Build history of the part. All positions in model axes, mm. A direction names the side the tool comes from. Give positions to 0.01 mm unless a question says otherwise; leave off trailing zeros. Write each loop counter-clockwise with the first axis right and the second up, starting at its lowest first coordinate (ties: lowest second). Pieces come first, ordered by that corner, then holes. Notation, with made-up numbers: (79, 47.5) -> (106, 47.5) arc R21 cw to (106, 59.5) -> close; hole circle Ø4 at (48, -3.75). An arc over 180 degrees is marked (long way). Put each result on its own line as item: value.
from build123d import *

# Parameters (mm, degrees)
F0_R      = 41
F0_R_2    = 8
F2_DEPTH  = 5
F5_DEPTH  = 5.001
F7_DEPTH  = 5.001
F9_DEPTH  = 5.001
F11_DEPTH = 5.001
F13_DEPTH = 5.001
F15_DEPTH = 25
F16_R     = 8
F17_DEPTH = 5.001
F19_DEPTH = 5.001
F21_DEPTH = 5.001
F22_R     = 8
F23_DEPTH = 5.001
F24_R     = 8
F25_DEPTH = 5.001
F26_R     = 8
F27_DEPTH = 5.001
F28_R     = 19.931343
F29_DEPTH = 5.001
F30_R     = 19.962779
F31_DEPTH = 5.001
F32_R     = 19.962779
F33_DEPTH = 5.001
F34_R     = 19.931343
F35_DEPTH = 5.001


with BuildPart() as f2:
    # F0 (on Top) → F2 (new body)
    with BuildSketch(Plane.XY):
        with Locations((-41.447371, -163.815796)):
            Circle(F0_R)
        with Locations((-41.447371, -163.815796)):
            Circle(F0_R_2, mode=Mode.SUBTRACT)
    extrude(amount=F2_DEPTH)

    # F4 (on face) → F5 (cut, through all)
    with BuildSketch(Plane.XY.offset(5)):
        Polygon((-38.297371, -151.997143), (-38.297371, -148.359836), (-41.447371, -146.541183), (-44.597371, -148.359836), (-44.597371, -151.997143), (-41.447371, -153.815796), align=None)
    extrude(amount=-F5_DEPTH, mode=Mode.SUBTRACT)

    # F6 (on face) → F7 (cut, through all)
    with BuildSketch(Plane.XY.offset(5)):
        Polygon((-37.747371, -142.904987), (-37.747371, -138.632595), (-41.447371, -136.496399), (-45.147371, -138.632595), (-45.147371, -142.904987), (-41.447371, -145.041183), align=None)
    extrude(amount=-F7_DEPTH, mode=Mode.SUBTRACT)

    # F8 (on face) → F9 (cut, through all)
    with BuildSketch(Plane.XY.offset(5)):
        Polygon((-47.747371, -131.359092), (-41.447371, -134.996399), (-35.147371, -131.359092), (-35.147371, -124.084479), (-41.447371, -120.447172), (-47.747371, -124.084479), align=None)
    extrude(amount=-F9_DEPTH, mode=Mode.SUBTRACT)

    # F10 (on face) → F11 (cut, through all)
    with BuildSketch(Plane.XY):
        Polygon((-38.347371, -175.605582), (-41.447371, -173.815796), (-44.547371, -175.605582), (-44.547371, -179.185154), (-41.447371, -180.97494), (-38.347371, -179.185154), align=None)
    extrude(amount=F11_DEPTH, mode=Mode.SUBTRACT)

    # F12 (on face) → F13 (cut, through all)
    with BuildSketch(Plane.XY):
        Polygon((-37.747371, -184.611136), (-41.447371, -182.47494), (-45.147371, -184.611136), (-45.147371, -188.883528), (-41.447371, -191.019724), (-37.747371, -188.883528), align=None)
    extrude(amount=F13_DEPTH, mode=Mode.SUBTRACT)

    # F14 (on face) → F15 (cut)
    with BuildSketch(Plane.XY):
        with BuildLine():
            Line((-35.097371, -196.185898), (-41.447371, -192.519724))
            Line((-41.447371, -192.519724), (-47.797371, -196.185898))
            Line((-47.797371, -196.185898), (-47.797371, -203.518246))
            Line((-47.797371, -203.518246), (-45.986492, -204.563758))
            ThreePointArc((-45.986492, -204.563758), (-41.447371, -204.815796), (-36.908251, -204.563758))
            Line((-36.908251, -204.563758), (-35.097371, -203.518246))
            Line((-35.097371, -203.518246), (-35.097371, -196.185898))
        make_face()
    extrude(amount=F15_DEPTH, mode=Mode.SUBTRACT)

    # F16 (on face) → F17 (cut, through all)
    with BuildSketch(Plane.XY):
        with Locations((-41.447371, -163.815796)):
            Circle(F16_R)
        Polygon((-24.288228, -163.815796), (-26.078014, -160.715796), (-29.657585, -160.715796), (-31.447371, -163.815796), align=None)
        Polygon((-26.078014, -166.915796), (-24.288228, -163.815796), (-31.447371, -163.815796), (-29.657585, -166.915796), align=None)
    extrude(amount=F17_DEPTH, mode=Mode.SUBTRACT)

    # F18 (on face) → F19 (cut, through all)
    with BuildSketch(Plane.XY):
        Polygon((-15.87964, -160.115796), (-20.152032, -160.115796), (-22.288228, -163.815796), (-20.152032, -167.515796), (-15.87964, -167.515796), (-13.743444, -163.815796), align=None)
    extrude(amount=F19_DEPTH, mode=Mode.SUBTRACT)

    # F20 (on face) → F21 (cut, through all)
    with BuildSketch(Plane.XY):
        with BuildLine():
            Line((-0.837825, -158.170907), (-1.244921, -157.465796))
            Line((-1.244921, -157.465796), (-8.57727, -157.465796))
            Line((-8.57727, -157.465796), (-12.243444, -163.815796))
            Line((-12.243444, -163.815796), (-8.57727, -170.165796))
            Line((-8.57727, -170.165796), (-1.244921, -170.165796))
            Line((-1.244921, -170.165796), (-0.837825, -169.460685))
            ThreePointArc((-0.837825, -169.460685), (-0.545101, -166.644985), (-0.447371, -163.815796))
            ThreePointArc((-0.447371, -163.815796), (-0.545101, -160.986608), (-0.837825, -158.170907))
        make_face()
    extrude(amount=F21_DEPTH, mode=Mode.SUBTRACT)

    # F22 (on face) → F23 (cut, through all)
    with BuildSketch(Plane.XY.offset(5)):
        Polygon((-53.237157, -160.715796), (-56.816729, -160.715796), (-58.606515, -163.815796), (-56.816729, -166.915796), (-53.237157, -166.915796), (-51.447371, -163.815796), align=None)
        with Locations((-41.447371, -163.815796)):
            Circle(F22_R)
    extrude(amount=-F23_DEPTH, mode=Mode.SUBTRACT)

    # F24 (on face) → F25 (cut, through all)
    with BuildSketch(Plane.XY.offset(5)):
        Polygon((-60.106515, -163.815796), (-62.242711, -160.115796), (-66.515103, -160.115796), (-68.651299, -163.815796), (-66.515103, -167.515796), (-62.242711, -167.515796), align=None)
        with Locations((-41.447371, -163.815796)):
            Circle(F24_R)
    extrude(amount=-F25_DEPTH, mode=Mode.SUBTRACT)

    # F26 (on face) → F27 (cut, through all)
    with BuildSketch(Plane.XY.offset(5)):
        Polygon((-85.315995, -163.815796), (-81.649821, -170.165796), (-74.317473, -170.165796), (-70.651299, -163.815796), (-74.317473, -157.465796), (-81.649821, -157.465796), align=None)
        with Locations((-41.447371, -163.815796)):
            Circle(F26_R)
    extrude(amount=-F27_DEPTH, mode=Mode.SUBTRACT)

    # F28 (on face) → F29 (cut, through all)
    with BuildSketch(Plane.XY.offset(5)):
        with Locations((-70.473262, -192.772621)):
            Circle(F28_R)
    extrude(amount=-F29_DEPTH, mode=Mode.SUBTRACT)

    # F30 (on face) → F31 (cut, through all)
    with BuildSketch(Plane.XY.offset(5)):
        with Locations((-70.446051, -134.831722)):
            Circle(F30_R)
    extrude(amount=-F31_DEPTH, mode=Mode.SUBTRACT)

    # F32 (on face) → F33 (cut, through all)
    with BuildSketch(Plane.XY.offset(5)):
        with Locations((-12.448691, -134.831722)):
            Circle(F32_R)
    extrude(amount=-F33_DEPTH, mode=Mode.SUBTRACT)

    # F34 (on face) → F35 (cut, through all)
    with BuildSketch(Plane.XY.offset(5)):
        with Locations((-12.421481, -192.772621)):
            Circle(F34_R)
    extrude(amount=-F35_DEPTH, mode=Mode.SUBTRACT)


solid = f2.part
1) Tool access for faces 1 (the flat face through (-39.88, -174.72, 2.46)), 2 (the cylindrical face through (-49.637, -123.642, 2.465)): list every direction of +Z, -Z, +X, -X, +Y, -Y with a clear straight run to the whole face (end or side of a thin tool).
Filled sheet:
face 1: +Z, -Z
face 2: +Z, -Z, -X, +Y
2) Pin check, flat tips, straight feed: pin 1 (1.8 mm diameter, centred on y = -176.5, z = 2, fed in from +X); pin 2 (1.8 mm diameter, centred on x = -27.5, z = 2.5, fed in from -Y); pin 3 (2 mm diameter, centred on x = -63.5, z = 2, fed in from +Y). Stop position of each tip, or through.
Filled sheet:
pin 1: x = -2.18
pin 2: y = -180.86
pin 3: y = -153.14
3) Wall check: L1, parallel to X at y = -164, z = 3.75; L2, parallel to Y at x = -39.5, z = 1.25; L3, parallel to Y at x = -34.5, z = 2.95. Give the ranges that are in metal, low to high.
Filled sheet:
L1: -70.76 to -68.54, -60.21 to -58.5, -51.55 to -49.45, -33.45 to -31.34, -24.39 to -22.18, -13.85 to -12.14
L2: -193.64 to -189.9, -183.6 to -179.85, -174.94 to -171.58, -156.06 to -152.69, -147.67 to -143.92, -137.62 to -133.87
L3: -204.22 to -167.78, -159.85 to -123.41
4) Pull direction X, two halves, no side cores. Call faces 3 (the cylindrical face through (-49.775, -203.961, 2.465)), 4 (the cylindrical face through (-33.22, -203.98, 2.46)), 5 (the flat face through (-18, -167.516, 2)): released by +X, released by -X, zero draft, split by the parting line, or undercut.
Filled sheet:
face 3: released by -X
face 4: released by +X
face 5: undercut
5) Slice it at A-A (x = -77). Write the cut outline in (y, z), plus the area to 3 significant figures.
Filled sheet:
outline: (-173.94, 0) -> (-170.17, 0) -> (-170.17, 5) -> (-173.94, 5) -> close; (-157.47, 0) -> (-153.69, 0) -> (-153.69, 5) -> (-157.47, 5) -> close
area: 37.8 mm2
6) Slice it at B-B (z = 1.85). Give the number of separate pieces and of enclosed holes in the cut face, plus the area to 3 significant figures.
Filled sheet:
separate pieces: 1
enclosed holes: 9
area: 2,010 mm2
